Design review of the part shown in the three views and the two pictorial views. Dimensions are in mm from the part's minimum x, y and z. Round coordinates to 2 decimals unless told otherwise and drop trailing zeros. Write each loop counter-clockwise with the first axis right and the second up, starting at its lowest first coordinate (ties: lowest second). Pieces come first, ordered by that corner, then holes. Notation, with made-up numbers: (17.5, 46) -> (74.5, 46) arc R24 cw to (74.5, 58) -> close; hole circle Ø3 at (-17.5, 67.25). An arc over 180 degrees is marked (long way). Answer as a JSON object with one key per item and string values. Group by question number.
1) We need section A-A, the plane z = 3.55. Write out the cut boundary in (x, y) (3 decimals), then the cut area to 3 significant figures.
2) We need section C-C, the plane x = 9. Write out the cut boundary in (y, z).
3) Insertion check: pin 1 Ø1.5 at (y, z) = (113, 3) entering from +X. The pin has a flat end and moves straight along its axis. Give the tip position at first contact, or say it passes through.
4) We need section B-B, the plane y = 108. Write out the cut boundary in (x, z).
5) To check wall thickness, follow probe 1 along X at (y, z) = (120, 1.35); probe 2 along Y at (x, z) = (17, 4.1); probe 3 along X at (y, z) = (84.5, 2.95). State the ranges of each line that lie inside material, in increasing order. Write a range as [from, to].
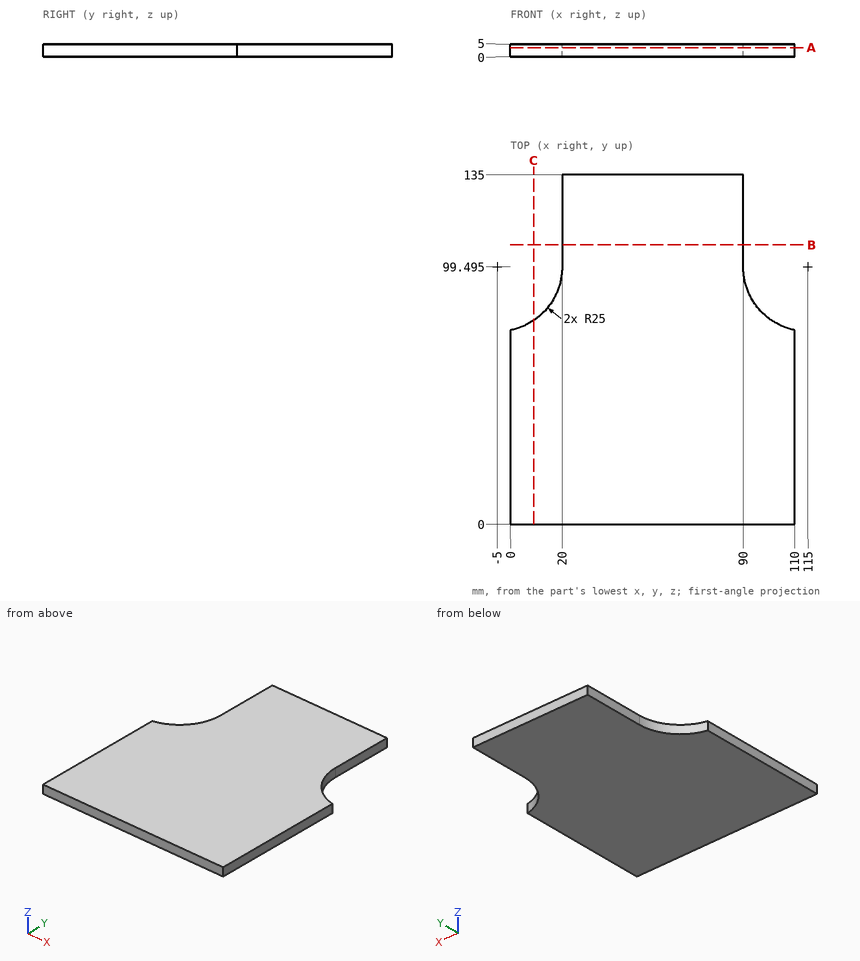
Here are the results:
{
 "1": {"outline": "(0, 0) -> (110, 0) -> (110, 75) arc R25 cw to (90, 99.495) -> (90, 135) -> (20, 135) -> (20, 99.495) arc R25 cw to (0, 75) -> close", "area": "12,700 mm^2"},
 "2": {"outline": "(0, 0) -> (78.78, 0) -> (78.78, 5) -> (0, 5) -> close"},
 "3": {"pin 1": "stops at x = 90"},
 "4": {"outline": "(20, 0) -> (90, 0) -> (90, 5) -> (20, 5) -> close"},
 "5": {"probe 1": "x = [20, 90]", "probe 2": "y = [0, 87.62]", "probe 3": "x = [15, 95]"}
}
